Job drawing, mm, ordinate dimensions from the low corner. One solid piece. Give positions to 0.01 mm unless a question says otherwise; leave off trailing zeros. Order: outer loops, then holes, each group sorted by start corner. A loop starts at its lowest first (then second) coordinate and runs counter-clockwise, first axis right, second up.
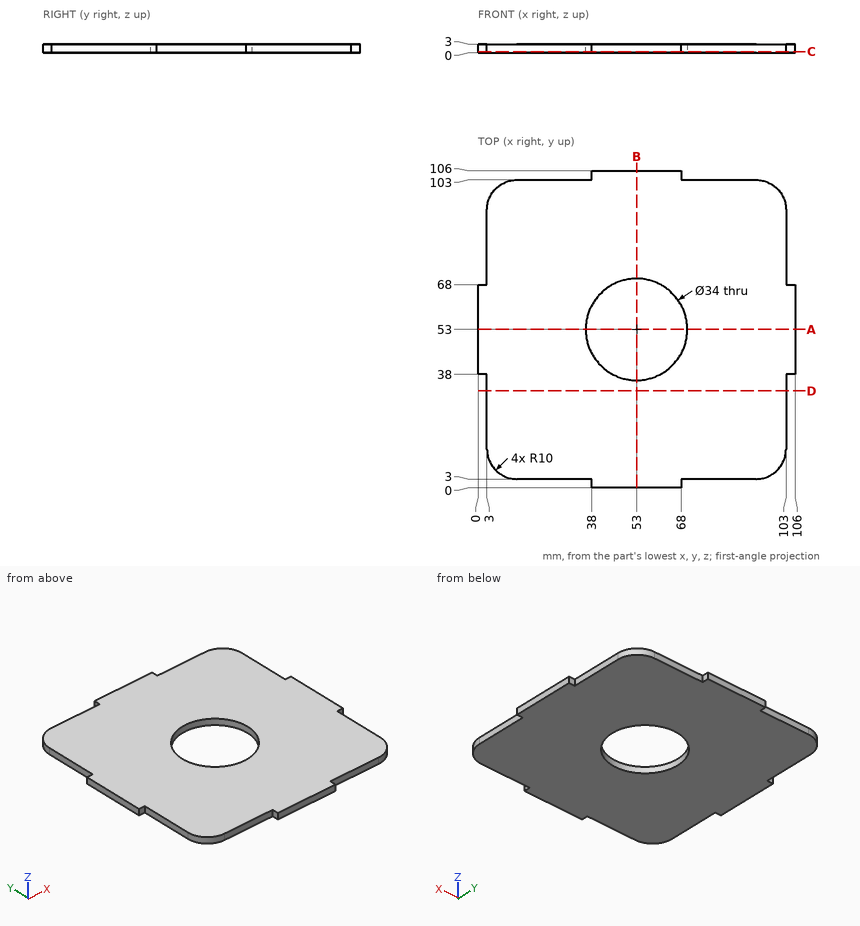
Item 1: Band-saw the part on D-D on y = 32.5. List the corners of the cut face in (x, z), plus the area to 3 significant figures.
Item 2: Drop flat-ended pins along their axis: P1, Ø0.9, axis at x = 104, z = 1.5, coming from the +Y side; P2, Ø0.9, axis at y = 1, z = 1.5, coming from the +X side; P3, Ø1.5, axis at y = 104.5, z = 2, coming from the -X side. Give the stop position or say it passes through.
Item 3: Drill centre lines: probe 1 along Y at (x, z) = (53, 2.1); probe 2 along X at (y, z) = (52, 0.95); probe 3 along X at (y, z) = (28, 1.9). Where is each one in solid material? Low to high.
Item 4: Band-saw the part on A-A on y = 53. List the corners of the cut face in (x, z), plus the area to 3 significant figures.
Item 5: Band-saw the part on C-C on z = 0.45. List the corners of the cut face in (x, y), plus the area to 3 significant figures.
Working result:
1. outline: (3, 0) - (103, 0) - (103, 3) - (3, 3) - close
1. area: 300 mm2
2. P1: stops at y = 68
2. P2: stops at x = 68
2. P3: stops at x = 38
3. probe 1: y = 0 to 36, 70 to 106
3. probe 2: x = 0 to 36.03, 69.97 to 106
3. probe 3: x = 3 to 103
4. outline: (0, 0) - (36, 0) - (36, 3) - (0, 3) - close; (70, 0) - (106, 0) - (106, 3) - (70, 3) - close
4. area: 216 mm2
5. outline: (0, 38) - (3, 38) - (3, 13) arc R10 ccw to (13, 3) - (38, 3) - (38, 0) - (68, 0) - (68, 3) - (93, 3) arc R10 ccw to (103, 13) - (103, 38) - (106, 38) - (106, 68) - (103, 68) - (103, 93) arc R10 ccw to (93, 103) - (68, 103) - (68, 106) - (38, 106) - (38, 103) - (13, 103) arc R10 ccw to (3, 93) - (3, 68) - (0, 68) - close; hole circle Ø34 at (53, 53)
5. area: 9,370 mm2
